Verification items for the finished model (mm, model axes). A direction names the side the tool comes from. Round coordinates to 2 decimals unless told otherwise and drop trailing zeros. Write each loop counter-clockwise with the first axis right and the second up, starting at its lowest first coordinate (ties: lowest second). Pieces come first, ordered by that corner, then holes. Notation, with made-up numbers: M -38,71 L 11,71 A34 ccw 11,103 Z; hole C 77,57 d2. An arc over 180 degrees is marked long. One line per item, written item: value. Start each with the question number.
Item 1: Gauge pin test, flat ends, axial feed: pin 1 (10 mm diameter, centred on x = -6.5, z = -8, fed in from -Y); pin 2 (1.6 mm diameter, centred on x = 13.5, y = -0.5, fed in from -Z); pin 3 (2 mm diameter, centred on y = 1.5, z = 9, fed in from -X). Record the tip position at first contact, or that the pin passes through.
Item 2: Section check D-D, the plane y = 1.5. State how many separate pieces and enclosed holes the cut face has, then the cut area to 3 significant figures.
Item 3: Section check B-B, the plane z = -9.25. Record the cut outline in (x, y).
Item 4: Tool access check on faces 4 (the face through (5.1, 1.3, -4.1)), 5 (the face through (-12.5, -2, 0)), 6 (the face through (9, 1, 13)), 7 (the face through (-13.5, 1, -9)). Record the directions out of +Z, -Z, +X, -X, +Y, -Y that give a thin tool (end or side, any length) a straight path to the whole face; none if there is none.
Item 5: Draft check along Z on faces 1 (the face through (-6.5, 1, 7)), 2 (the face through (0, -1, 14)), 3 (the face through (0, -4.5, 13)). Enter one of: +Z half, -Z half, draft (parallel to the pull), parting line (faces both ways), or undercut.
Item 6: Section check C-C, the plane z = 0.25. Record the cut outline in (x, y), then the cut area to 3 significant figures.
Item 7: Section check A-A, the plane y = -1.5. Record the cut outline in (x, z), then the cut area to 3 significant figures.
Item 8: Thickness scan on probe 1 along X at (y, z) = (0.25, 5.75); probe 2 along X at (y, z) = (-0.5, 0.5); probe 3 along X at (y, z) = (0.5, -9.5). Record the ranges inside material, lowest first. Write a range as from..to.
from build123d import *

# Parameters (mm, degrees)
BOSS_EXTRUDE1_DEPTH      = 2.5
BOSS_EXTRUDE2_DEPTH      = 4.5
BOSS_EXTRUDE2_DEPTH_BACK = 2.5
SKETCH2_W                = 2
SKETCH2_H                = 14.9
SKETCH2_W_2              = 14.9
SKETCH2_H_2              = 2
CUT_EXTRUDE1_DEPTH       = 10


with BuildPart() as part:
    # Sketch1 → Boss-Extrude1 (new body)
    with BuildSketch(Plane(origin=(0, 0, 0), x_dir=(1, 0, 0), z_dir=(0, 1, 0))):
        with BuildLine():
            Line((-10.5, -13), (10.5, -13))
            ThreePointArc((10.5, -13), (12.621320344, -12.121320344), (13.5, -10))
            Line((13.5, -10), (13.5, 10))
            ThreePointArc((13.5, 10), (12.621320344, 12.121320344), (10.5, 13))
            Line((10.5, 13), (-10.5, 13))
            ThreePointArc((-10.5, 13), (-12.621320344, 12.121320344), (-13.5, 10))
            Line((-13.5, 10), (-13.5, -10))
            ThreePointArc((-13.5, -10), (-12.621320344, -12.121320344), (-10.5, -13))
        make_face()
    extrude(amount=BOSS_EXTRUDE1_DEPTH)

    # Sketch2 → Boss-Extrude2 (add, two sides: drawn at the far end of the back side and taken through both)
    with BuildSketch(Plane.XZ.offset(-BOSS_EXTRUDE2_DEPTH_BACK)):
        with Locations((-13.5, 0)):
            Rectangle(SKETCH2_W, SKETCH2_H)
        with Locations((13.5, 0)):
            Rectangle(SKETCH2_W, SKETCH2_H)
        with Locations((0, 13)):
            Rectangle(SKETCH2_W_2, SKETCH2_H_2)
    extrude(amount=BOSS_EXTRUDE2_DEPTH + BOSS_EXTRUDE2_DEPTH_BACK)

    # Sketch3 → Cut-Extrude1 (cut)
    with BuildSketch(Plane(origin=(0, 2.5, 0), x_dir=(1, 0, 0), z_dir=(0, 1, 0))):
        Polygon((1, -4.907477288), (3.75, -3.319764048), (6.5, -4.907477288), (6.5, -8.082903769), (3.75, -9.670617009), (1, -8.082903769), align=None)
        Polygon((-3.75, 3.319764048), (-1, 4.907477288), (-1, 8.082903769), (-3.75, 9.670617009), (-6.5, 8.082903769), (-6.5, 4.907477288), align=None)
        Polygon((-7.5, -3.175426481), (-4.75, -1.58771324), (-4.75, 1.58771324), (-7.5, 3.175426481), (-10.25, 1.58771324), (-10.25, -1.58771324), align=None)
        Polygon((7.5, -3.175426481), (10.25, -1.58771324), (10.25, 1.58771324), (7.5, 3.175426481), (4.75, 1.58771324), (4.75, -1.58771324), align=None)
        Polygon((3.75, 3.319764048), (6.5, 4.907477288), (6.5, 8.082903769), (3.75, 9.670617009), (1, 8.082903769), (1, 4.907477288), align=None)
        Polygon((-6.5, -4.907477288), (-3.75, -3.319764048), (-1, -4.907477288), (-1, -8.082903769), (-3.75, -9.670617009), (-6.5, -8.082903769), align=None)
    extrude(amount=-CUT_EXTRUDE1_DEPTH, mode=Mode.SUBTRACT)


solid = part.part
Response values:
1. pin 1: stops at y = 0
1. pin 2: stops at z = -11.83
1. pin 3: stops at x = -13.5
2. separate pieces: 1
2. enclosed holes: 6
2. area: 582 mm2
3. outline: M -13.5,0 L -4.48,0 L -4.48,2.5 L -13.5,2.5 Z; M -3.02,0 L 3.02,0 L 3.02,2.5 L -3.02,2.5 Z; M 4.48,0 L 13.5,0 L 13.5,2.5 L 4.48,2.5 Z
4. face 4: +Y, -Y
4. face 5: +Z, -Z, -Y
4. face 6: +Z, +X, +Y, -Y
4. face 7: -Z, -X, +Y, -Y
5. face 1: undercut
5. face 2: +Z half
5. face 3: draft
6. outline: M -14.5,-4.5 L -12.5,-4.5 L -12.5,0 L -10.25,0 L -10.25,2.5 L -14.5,2.5 Z; M -4.75,0 L 4.75,0 L 4.75,2.5 L -4.75,2.5 Z; M 10.25,0 L 12.5,0 L 12.5,-4.5 L 14.5,-4.5 L 14.5,2.5 L 10.25,2.5 Z
6. area: 63.0 mm2
7. outline: M -14.5,-7.45 L -12.5,-7.45 L -12.5,7.45 L -14.5,7.45 Z; M -7.45,12 L 7.45,12 L 7.45,14 L -7.45,14 Z; M 12.5,-7.45 L 14.5,-7.45 L 14.5,7.45 L 12.5,7.45 Z
7. area: 89.4 mm2
8. probe 1: x = -14.5..-6.5, -1..1, 6.5..14.5
8. probe 2: x = -14.5..-12.5, 12.5..14.5
8. probe 3: x = -13.5..-4.05, -3.45..3.45, 4.05..13.5
